Verification items for the finished model (mm, model axes). A direction names the side the tool comes from. Give positions to 0.01 mm unless a question says otherwise; leave off trailing zeros. Write each loop counter-clockwise with the first axis right and the second up, starting at its lowest first coordinate (ties: lowest second). Pieces come first, ordered by that corner, then holes. Notation, with made-up numbers: (-13.5, 18) - (10.5, 18) arc R30 ccw to (10.5, 44) - close; hole circle Ø7 at (73, 53). An arc over 180 degrees is marked (long way). Put each result on its own line as item: value.
from build123d import *

# Parameters (mm, degrees)
SKETCH2_W           = 17
SKETCH2_H           = 35
BOSS_EXTRUDE1_DEPTH = 40
SKETCH3_W           = 12.1
SKETCH3_H           = 32.32
CUT_EXTRUDE1_DEPTH  = 10.73
SKETCH4_W           = 12.5
SKETCH4_H           = 28.5
CUT_EXTRUDE2_DEPTH  = 17
SKETCH6_W           = 9
SKETCH6_H           = 6.5
CUT_EXTRUDE3_DEPTH  = 17
SKETCH7_W           = 10.843475329
SKETCH7_H           = 35
CUT_EXTRUDE4_DEPTH  = 56.803225713


with BuildPart() as part:
    # Sketch2 → Boss-Extrude1 (new body)
    with BuildSketch(Plane.XY):
        with Locations((-8.5, 17.5)):
            Rectangle(SKETCH2_W, SKETCH2_H)
    extrude(amount=BOSS_EXTRUDE1_DEPTH)

    # Sketch3 → Cut-Extrude1 (cut)
    with BuildSketch(Plane.XY.offset(40)):
        with Locations((-8.5, 17.5)):
            Rectangle(SKETCH3_W, SKETCH3_H)
    extrude(amount=-CUT_EXTRUDE1_DEPTH, mode=Mode.SUBTRACT)

    # Sketch4 → Cut-Extrude2 (cut)
    with BuildSketch(Plane.XY.offset(29.27)):
        with Locations((-8.5, 17.5)):
            Rectangle(SKETCH4_W, SKETCH4_H)
    extrude(amount=-CUT_EXTRUDE2_DEPTH, mode=Mode.SUBTRACT)

    # Sketch6 → Cut-Extrude3 (cut)
    with BuildSketch(Plane(origin=(0, 3.25, 0), x_dir=(1, 0, 0), z_dir=(0, 1, 0))):
        with Locations((-8.5, -17.044771265)):
            Rectangle(SKETCH6_W, SKETCH6_H)
    extrude(amount=-CUT_EXTRUDE3_DEPTH, mode=Mode.SUBTRACT)

    # Sketch7 → Cut-Extrude4 (cut, through all)
    with BuildSketch(Plane.ZY.offset(17)):
        with Locations((5.421737665, 17.5)):
            Rectangle(SKETCH7_W, SKETCH7_H)
    extrude(amount=-CUT_EXTRUDE4_DEPTH, mode=Mode.SUBTRACT)


solid = part.part
Q1. Go/stop test with flat-tipped pins: pin 1 Ø1.5 at (x, y) = (-8.5, 32.5) entering from +Z; pin 2 Ø6 at (x, y) = (-7, 14) entering from +Z. Record where each tip stops, or that it passes through.
Answers follow:
pin 1: stops at z = 29.27
pin 2: stops at z = 12.27
Q2. Section check A-A, the plane z = 22.75. Record the cut outline in (x, y).
Answers follow:
outline: (-17, 0) - (0, 0) - (0, 35) - (-17, 35) - close; hole (-14.75, 3.25) - (-2.25, 3.25) - (-2.25, 31.75) - (-14.75, 31.75) - close
Q3. Section check B-B, the plane x = -8.75. Record the cut outline in (y, z), plus the area to 3 significant figures.
Answers follow:
outline: (0, 10.84) - (35, 10.84) - (35, 40) - (33.66, 40) - (33.66, 29.27) - (31.75, 29.27) - (31.75, 12.27) - (3.25, 12.27) - (3.25, 13.79) - (0, 13.79) - close; (0, 20.29) - (3.25, 20.29) - (3.25, 29.27) - (1.34, 29.27) - (1.34, 40) - (0, 40) - close
area: 168 mm2
Q4. Release check for a two-part mould opening along X. For faces 4 (the face through (0, 17, 25)), 5 (the face through (-2.25, 17, 21)), 6 (the face through (-9, 17, 10.843)) record: released by +X, released by -X, zero draft, split by the parting line, or undercut.
Answers follow:
face 4: released by +X
face 5: undercut
face 6: zero draft
Q5. Section check D-D, the plane x = -13.5. Record the cut outline in (y, z), plus the area to 3 significant figures.
Answers follow:
outline: (0, 10.84) - (35, 10.84) - (35, 40) - (33.66, 40) - (33.66, 29.27) - (31.75, 29.27) - (31.75, 12.27) - (3.25, 12.27) - (3.25, 29.27) - (1.34, 29.27) - (1.34, 40) - (0, 40) - close
area: 189 mm2
Q6. Scan lines: line 1 along X through (y, z) = (16, 31); line 2 along Y through (x, z) = (-13.25, 32.25); line 3 along X through (y, z) = (19, 16.25). Record each from-to range of solid material in increasing order.
Answers follow:
line 1: x = -17 to -14.55, -2.45 to 0
line 2: y = 0 to 1.34, 33.66 to 35
line 3: x = -17 to -14.75, -2.25 to 0
Q7. Section check C-C, the plane y = 28. Record the cut outline in (x, z).
Answers follow:
outline: (-17, 10.84) - (0, 10.84) - (0, 40) - (-2.45, 40) - (-2.45, 29.27) - (-2.25, 29.27) - (-2.25, 12.27) - (-14.75, 12.27) - (-14.75, 29.27) - (-14.55, 29.27) - (-14.55, 40) - (-17, 40) - close
Q8. Set-up check for faces 1 (the face through (-9, 33, 29.27)), 2 (the face through (-9, 0, 25)), 3 (the face through (-9, 2, 13.795)): record each of +Z, -Z, +X, -X, +Y, -Y from which the full face is reachable in a straight line by a thin tool's end or side.
Answers follow:
face 1: +Z
face 2: +Z, -Z, +X, -X, -Y
face 3: -Y
